Autodesk Inventor part; units mm, degrees
ref_plane "YZ Plane" through (0, 0, 0) normal (1, 0, 0) x (0, 1, 0)
ref_plane "XZ Plane" through (0, 0, 0) normal (0, 1, 0) x (-1, 0, 0)
ref_plane "XY Plane" through (0, 0, 0) normal (0, 0, 1) x (1, 0, 0)
sketch "Esboço1" plane through (0, 0, 0) normal (0, 0, 1) x (1, 0, 0)
  line L0 (0, -20.4) -> (0, 10.4) construction
  line L1 (-3.6, 0) -> (0.6, 0) construction
  line L2 (0, -16) -> (-2, -16)
  line L3 (-2, -16) -> (-2, 0)
  line L4 (-2, 0) -> (-3, 0)
  line L5 (-3, 0) -> (-3, 4)
  line L6 (-3, 4) -> (-1.25, 4)
  line L7 (-1.25, 4) -> (-1.25, 6)
  line L8 (-1.25, 6) -> (0, 6)
  line L9 (0, 6) -> (0, -16)
  line L10 (-0.5, 6) -> (-1.25, 5.25)
  line L11 (-2, -15.5) -> (-1.5, -16)
  line L12 (-3, 3.8) -> (-2.8, 4)
  line L13 (-3, 2) -> (0, 2) construction
  line L14 (-3, 0.2) -> (-2.8, 0)
  line L15 (-2, -2) -> (-1.75, -2)
  line L16 (-1.75, -2) -> (-1.75, 0)
  line L17 (-1.75, 0) -> (-2, 0)
  line L18 (-2, 0) -> (-2, -2)
  line L19 (-1.75, -2) -> (-2, -2.25)
  point P0 (0, 0)
  dimension "d0" = 2
  dimension "d1" = 6
  dimension "d2" = 2.5
  dimension "d3" = 0.75
  dimension "d4" = 0.75
  dimension "d5" = 4
  dimension "d6" = 16
  dimension "d7" = 22
  dimension "d8" = 4
  dimension "d9" = 0.5
  dimension "d10" = 0.5
  dimension "d12" = 0.2
  dimension "d13" = 0.2
  dimension "d16" = 3.5
  dimension "d17" = 2
  dimension "d18" = 0.25
  dimension "d19" = 0.25
revolve "Revolução1" add sketch "Esboço1" angle 360 about axis through (0, -10, 0) along (0, 1, 0) contours L2 L11 L3 L19 L16 L17 L4 L14 L5 L12 L6 L7 L10 L8 L9
thread "Rosca1"
equation "\"d4\" = d3"
equation "\"d10\" = d9"
equation "\"d18\" = d19"
properties part number "GRJ-03-119" material "Aço SAE 1045"
Verification items for the finished model (mm, model axes). A direction names the side the tool comes from. Round coordinates to 2 decimals unless told otherwise and drop trailing zeros. Loops run counter-clockwise (first coordinate to the right, second up) from the corner with the lowest first, then second, coordinate; pieces in that order, holes last. Notation, with made-up numbers: (73.25, -34.5) - (81.25, -34.5) arc R23 ccw to (81.25, 0.5) - close; hole circle Ø5 at (69, -5). An arc over 180 degrees is marked (long way). Use a Markdown table: item, result. Add a question column.
1. Section check D-D, the plane y = -5.75. Record the boundary of the cut face in (x, z).
2. Section check B-B, the plane z = 0. Record the boundary of the cut face in (x, y), plus the area to 3 significant figures.
3. Access from +Z, -Z, +X, -X, +Y, -Y to the whole of each face (thin tool, end or side, straight path). Record for faces 1 (the face through (0, 0, -2)), 2 (the face through (0.27, 4.63, -1.22)), 3 (the face through (0, -9, -2)).
4. Thickness scan on probe 1 along Y at (x, z) = (-0.4, 2.35); probe 2 along Z at (x, y) = (-0.05, -14); probe 3 along Y at (x, z) = (1.1, 1.4). Record the ranges inside material, lowest first. Write a range as [from, to].
5. Gauge pin test, flat ends, axial feed: pin 1 (2 mm diameter, centred on x = -2, y = -2.5, fed in from +Z); pin 2 (1 mm diameter, centred on x = -1.5, z = -0.5, fed in from +Y); pin 3 (3 mm diameter, centred on y = -9.5, z = 0.5, fed in from -X). Record the tip position at first contact, or that the pin passes through.
6. Section check A-A, the plane x = 0. Record the boundary of the cut face in (y, z), plus the area to 3 significant figures.
7. Section check C-C, the plane y = 4.5. Record the boundary of the cut face in (x, z).
Checks:
| question | item | result |
|---|---|---|
| 1 | outline | circle Ø4 at (0, 0) |
| 2 | outline | (-3, 0.2) - (-2.8, 0) - (-1.75, 0) - (-1.75, -2) - (-2, -2.25) - (-2, -15.5) - (-1.5, -16) - (1.5, -16) - (2, -15.5) - (2, -2.25) - (1.75, -2) - (1.75, 0) - (2.8, 0) - (3, 0.2) - (3, 3.8) - (2.8, 4) - (1.25, 4) - (1.25, 5.25) - (0.5, 6) - (-0.5, 6) - (-1.25, 5.25) - (-1.25, 4) - (-2.8, 4) - (-3, 3.8) - close |
| 2 | area | 91.0 mm^2 |
| 3 | face 1 | none |
| 3 | face 2 | +Y |
| 3 | face 3 | -Y |
| 4 | probe 1 | y = [0, 4] |
| 4 | probe 2 | z = [-2, 2] |
| 4 | probe 3 | y = [-15.72, -2.03], [0, 4] |
| 5 | pin 1 | stops at z = 1.73 |
| 5 | pin 2 | stops at y = 5.42 |
| 5 | pin 3 | stops at x = -2 |
| 6 | outline | (-16, -1.5) - (-15.5, -2) - (-2.25, -2) - (-2, -1.75) - (0, -1.75) - (0, -2.8) - (0.2, -3) - (3.8, -3) - (4, -2.8) - (4, -1.25) - (5.25, -1.25) - (6, -0.5) - (6, 0.5) - (5.25, 1.25) - (4, 1.25) - (4, 2.8) - (3.8, 3) - (0.2, 3) - (0, 2.8) - (0, 1.75) - (-2, 1.75) - (-2.25, 2) - (-15.5, 2) - (-16, 1.5) - close |
| 6 | area | 91.0 mm^2 |
| 7 | outline | circle Ø2.5 at (0, 0) |
